Could you check a few things on this drawing? It's one solid part, dimensions in mm from its lowest x, y, z. A direction names the side the tool comes from. Give positions to 0.01 mm unless a question says otherwise; leave off trailing zeros. Write each loop counter-clockwise with the first axis right and the second up, starting at its lowest first coordinate (ties: lowest second). Pieces come first, ordered by that corner, then holes. Notation, with made-up numbers: (80, -38) -> (89, -38) arc R34 cw to (89, -3) -> close; hole circle Ø2 at (-32, 2.5). An arc over 180 degrees is marked (long way). Answer as CSV lines item,"result". Start each with the question number.
1. On a 3-axis mill with a long thin cutter (end or side, diameter ignored), from which of +Z, -Z, +X, -X, +Y, -Y can I reach the whole of each face in a straight line? I mean the marked faces 4, 5 and 6. Say none if no direction works.
2. I need wall thicknesses on line 1 (X direction, y = 8, z = 2) (1 decimal); line 2 (Y direction, x = 2, z = 1.05) (1 decimal); line 3 (X direction, y = 4.75, z = 2.9) (1 decimal). Which ranges of each line are inside material? Lowest first, please. Write a range as [from, to].
3. If we section it at C-C on x = 6: Write out the boundary of the cut face in (y, z) (1 decimal).
4. I'm going to push flat-ended pins straight in: P1, Ø3, axis at y = 11, z = 3, coming from the -X side; P2, Ø0.8, axis at x = 3.5, z = 1.5, coming from the -Y side. Where does each tip first touch, or does it pass through?
5. If we section it at A-A on y = 6.5: Write out the boundary of the cut face in (x, z) (1 decimal).
6. If we mould it in two halves opening along X, with no side actions, what happens to the marked faces 1, 2 and 3? For each: pulls with the +X half, pulls with the -X half, needs draft (parallel to the pull), parting line crosses it, or undercut.
7. If we section it at B-B on z = 4.65: Write out the boundary of the cut face in (x, y) (1 decimal).
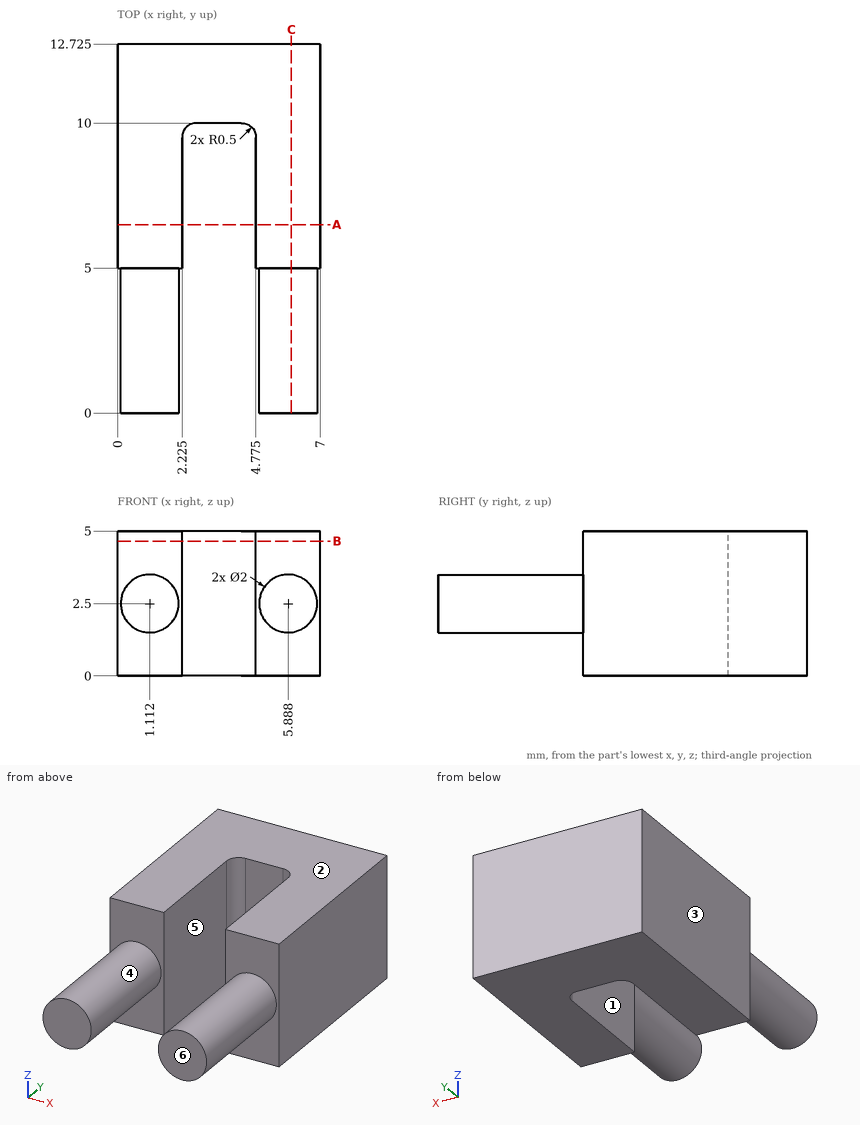
Computed values:
1,face 4,"-Y"
1,face 5,"+Z, -Z, -Y"
1,face 6,"+Z, -Z, +X, -X, -Y"
2,line 1,"x = [0, 2.2], [4.8, 7]"
2,line 2,"y = [5, 12.7]"
2,line 3,"x = [0.2, 2], [5, 6.8]"
3,outline,"(0, 1.5) -> (5, 1.5) -> (5, 0) -> (12.7, 0) -> (12.7, 5) -> (5, 5) -> (5, 3.5) -> (0, 3.5) -> close"
4,P1,"stops at x = 0"
4,P2,"stops at y = 10"
5,outline,"(0, 0) -> (2.2, 0) -> (2.2, 5) -> (0, 5) -> close; (4.8, 0) -> (7, 0) -> (7, 5) -> (4.8, 5) -> close"
6,face 1,"undercut"
6,face 2,"needs draft"
6,face 3,"pulls with the -X half"
7,outline,"(0, 5) -> (2.2, 5) -> (2.2, 9.5) arc R0.5 cw to (2.7, 10) -> (4.3, 10) arc R0.5 cw to (4.8, 9.5) -> (4.8, 5) -> (7, 5) -> (7, 12.7) -> (0, 12.7) -> close"
